```python
from build123d import *

# Parameters (mm, degrees)
SKETCH1_R                = 114.3
SKETCH1_R_2              = 96.8375
BOSS_EXTRUDE1_DEPTH      = 9.525
BOSS_EXTRUDE2_DEPTH      = 9.525
FILLET2_R                = 7.62
CIRPATTERN1_COUNT        = 6
FILLET2_OF_CIRPATTERN1_R = 7.62
F_1_4_CLEARANCE_HOLE1_D  = 6.7564
SKETCH2_R                = 2.38125
BOSS_EXTRUDE3_START      = -9.525
BOSS_EXTRUDE3_DEPTH      = 9.525
FILLET3_R                = 7.62
F_1_4_28_TAPPED_HOLE1_D  = 5.4102


with BuildPart() as part:
    # Sketch1 → Boss-Extrude1 (new body)
    with BuildSketch(Plane(origin=(0, 0, 0), x_dir=(1, 0, 0), z_dir=(0, 1, 0))):
        with Locations(Location((0, 0, 0), (0, 0, 90))):
            Circle(SKETCH1_R)
        with Locations(Location((0, 0, 0), (0, 0, 90))):
            Circle(SKETCH1_R_2, mode=Mode.SUBTRACT)
    extrude(amount=BOSS_EXTRUDE1_DEPTH)

    # Sketch3 → Boss-Extrude2 (add)
    with BuildSketch(Plane.XZ):
        with BuildLine():
            Line((95.930274374, -13.224366326), (82.55, -5.499261314))
            ThreePointArc((82.55, -5.499261314), (79.375, 0), (82.55, 5.499261314))
            Line((82.55, 5.499261314), (95.930274374, 13.224366326))
            ThreePointArc((95.930274374, 13.224366326), (96.8375, 0), (95.930274374, -13.224366326))
        make_face()
    boss_extrude2 = extrude(amount=-BOSS_EXTRUDE2_DEPTH)

    # Fillet2
    fillet2_edges = [part.edges().sort_by_distance(p)[0] for p in [
        (95.930274374, 4.7625, -13.224366326),
        (95.930274374, 4.7625, 13.224366326),
    ]]
    fillet(fillet2_edges, radius=FILLET2_R)

    # CirPattern1: Boss-Extrude2 ×6 about axis
    cirpattern1_axis = Axis((0, 0, 0), (0, 1, 0))
    for i in range(1, CIRPATTERN1_COUNT):
        add(boss_extrude2.rotate(cirpattern1_axis, i * 360 / CIRPATTERN1_COUNT))

    # Fillet2 of CirPattern1
    fillet2_of_cirpattern1_edges = [part.edges().sort_by_distance(p)[0] for p in [
        (36.5125, 4.7625, -89.690237763),
        (59.417774374, 4.7625, -76.465871437),
        (-59.417774374, 4.7625, -76.465871437),
        (-36.5125, 4.7625, -89.690237763),
        (-95.930274374, 4.7625, 13.224366326),
        (-95.930274374, 4.7625, -13.224366326),
        (-36.5125, 4.7625, 89.690237763),
        (-59.417774374, 4.7625, 76.465871437),
        (59.417774374, 4.7625, 76.465871437),
        (36.5125, 4.7625, 89.690237763),
    ]]
    fillet(fillet2_of_cirpattern1_edges, radius=FILLET2_OF_CIRPATTERN1_R)

    # 1/4 Clearance Hole1 (through all)
    with Locations(Plane(origin=(0, 0, 0), x_dir=(-1, 0, 0), z_dir=(0, -1, 0))):
        with Locations((-42.8625, 74.240027739), (42.8625, 74.240027739), (85.725, 0), (42.8625, -74.240027739), (-42.8625, -74.240027739), (-85.725, 0)):
            Hole(F_1_4_CLEARANCE_HOLE1_D / 2)

    # Sketch2 → Cut-Revolve1 (revolve, cut)
    with BuildSketch(Plane(origin=(0, 0, 0), x_dir=(0, 0, -1), z_dir=(1, 0, 0)), mode=Mode.PRIVATE) as cut_revolve1_sk:
        with Locations((-101.6, 10.795)):
            Circle(SKETCH2_R)
        with Locations((-101.6, -1.27)):
            Circle(SKETCH2_R)
    revolve(cut_revolve1_sk.sketch.rotate(Axis((0, 0, 0), (0, 1, 0)), 180), axis=Axis((0, 0, 0), (0, 1, 0)), mode=Mode.SUBTRACT)

    # Sketch7 → Boss-Extrude3 (add)
    with BuildSketch(Plane(origin=(0, 9.525, 0), x_dir=(1, 0, 0), z_dir=(0, 1, 0)).offset(BOSS_EXTRUDE3_START)):
        with BuildLine():
            Line((42.8625, -67.890027739), (25.4, -67.890027739))
            ThreePointArc((25.4, -67.890027739), (20.909871939, -69.749899679), (19.05, -74.240027739))
            Line((19.05, -74.240027739), (19.05, -94.94524162))
            ThreePointArc((19.05, -94.94524162), (25.259903299, -93.484965056), (31.360186833, -91.618994145))
            ThreePointArc((31.360186833, -91.618994145), (35.092023113, -88.840241596), (36.5125, -84.409630671))
            Line((36.5125, -84.409630671), (36.5125, -74.240027739))
            ThreePointArc((36.5125, -74.240027739), (38.372371939, -69.749899679), (42.8625, -67.890027739))
        make_face()
        with BuildLine():
            Line((-42.8625, -67.890027739), (-25.4, -67.890027739))
            ThreePointArc((-25.4, -67.890027739), (-20.909871939, -69.749899679), (-19.05, -74.240027739))
            Line((-19.05, -74.240027739), (-19.05, -94.94524162))
            ThreePointArc((-19.05, -94.94524162), (-25.259903299, -93.484965056), (-31.360186833, -91.618994145))
            ThreePointArc((-31.360186833, -91.618994145), (-35.092023113, -88.840241596), (-36.5125, -84.409630671))
            Line((-36.5125, -84.409630671), (-36.5125, -74.240027739))
            ThreePointArc((-36.5125, -74.240027739), (-38.372371939, -69.749899679), (-42.8625, -67.890027739))
        make_face()
    extrude(amount=BOSS_EXTRUDE3_DEPTH)

    # Fillet3
    fillet3_edges = [part.edges().sort_by_distance(p)[0] for p in [
        (19.05, 4.7625, 94.94524162),
        (-19.05, 4.7625, 94.94524162),
    ]]
    fillet(fillet3_edges, radius=FILLET3_R)

    # 1/4-28 Tapped Hole1 (through all)
    with Locations(Plane(origin=(0, 9.525, 0), x_dir=(1, 0, 0), z_dir=(0, 1, 0))):
        with Locations((25.4, -74.240027739), (-25.4, -74.240027739)):
            Hole(F_1_4_28_TAPPED_HOLE1_D / 2)


solid = part.part
```
Geometry check sheet. Reference: the model listing, model coordinates, mm. A direction names the side the tool comes from. Round coordinates to 2 decimals unless told otherwise and drop trailing zeros. Order: outer loops, then holes, each group sorted by start corner. A loop starts at its lowest first (then second) coordinate and runs counter-clockwise, first axis right, second up. Notation, with made-up numbers: (-27.75, 38) - (31.25, 38) arc R15 cw to (31.25, 56) - close; hole circle Ø5 at (27.5, 29). An arc over 180 degrees is marked (long way). Use a Markdown table: item, result. Add a question column.
(1) Sectioned sample at B-B, the plane y = 3.25. Count the separate pieces of the cut face and the enclosed holes in it, and give its area (3 significant figures).
(2) Tool access check on faces 4 (the cylindrical face through (35.053, 4.829, -88.894)), 5 (the flat face through (22, 0, 73)). Record the directions out of +Z, -Z, +X, -X, +Y, -Y that give a thin tool (end or side, any length) a straight path to the whole face; none if there is none.
(3) Sectioned sample at A-A, the plane z = 0. Enter the section's corners in (x, y) (1 decimal), and give its area (3 significant figures).
(4) Release check for a two-part mould opening along Z. For faces 1 (the flat face through (-85, 9.525, 60)), 2 (the cylindrical face through (-5.03, 4.7, 114.19)), 3 (the cylindrical face through (-35.13, 4.83, -88.79)) record: pulls with the +Z half, pulls with the -Z half, needs draft (parallel to the pull), parting line crosses it, or undercut.
(5) Depth check by flat-ended pin: pin 1 (1 mm diameter, centred on x = 80.5, y = 6.5, fed in from +Z); pin 2 (2 mm diameter, centred on x = -77, y = 7.5, fed in from -Z); pin 3 (3 mm diameter, centred on x = -34.5, y = 3, fed in from -Z). Enter the tip coordinate at first touch or a pass-through.
(6) Material ranges on line 1 along Z through (x, y) = (-0.5, 7.25); line 2 along X through (y, z) = (8.75, -50.5); line 3 along Z through (x, y) = (-8.5, 0.75), recorded low to high. Write a range as [from, to].
Answers below:
| question | item | result |
|---|---|---|
| 1 | separate pieces | 1 |
| 1 | enclosed holes | 9 |
| 1 | area | 14,000 mm² |
| 2 | face 4 | +Y, -Y |
| 2 | face 5 | +Z, -Z, +X, -X, -Y |
| 3 | outline | (-114.3, 0) - (-103.6, 0) arc R2.4 cw to (-99.6, 0) - (-89.1, 0) - (-89.1, 9.5) - (-99.6, 9.5) arc R2.4 cw to (-103.6, 9.5) - (-114.3, 9.5) - close; (-82.3, 0) - (-79.4, 0) - (-79.4, 9.5) - (-82.3, 9.5) - close; (79.4, 0) - (82.3, 0) - (82.3, 9.5) - (79.4, 9.5) - close; (89.1, 0) - (99.6, 0) arc R2.4 cw to (103.6, 0) - (114.3, 0) - (114.3, 9.5) - (103.6, 9.5) arc R2.4 cw to (99.6, 9.5) - (89.1, 9.5) - close |
| 3 | area | 524 mm² |
| 4 | face 1 | needs draft |
| 4 | face 2 | parting line crosses it |
| 4 | face 3 | undercut |
| 5 | pin 1 | z = 81.64 |
| 5 | pin 2 | z = -85.37 |
| 5 | pin 3 | z = -109.43 |
| 6 | line 1 | [-114.3, -96.84], [96.84, 114.3] |
| 6 | line 2 | [-102.54, -89.56], [-86.75, -82.63], [82.63, 86.75], [89.56, 102.54] |
| 6 | line 3 | [-113.98, -102.51], [-99.98, -96.46], [96.46, 99.98], [102.51, 113.98] |
